CAD build for the part. Positions are in the model's coordinates, mm. Face numbers are marked on the shaded views. A direction names the side the tool comes from. Round coordinates to 2 decimals unless told otherwise and drop trailing zeros. Loops run counter-clockwise (first coordinate to the right, second up) from the corner with the lowest first, then second, coordinate; pieces in that order, holes last. Notation, with made-up numbers: (-34, 5.25) - (19, 5.25) arc R22 ccw to (19, 40.25) - close; hole circle Ø4 at (-0.5, -26). An arc over 180 degrees is marked (long way). One line per question, with ' | ' between items.
```python
from build123d import *

# Parameters (mm, degrees)
BASPROSKE_W              = 6
BASPROSKE_H              = 11.25
TOOTHCUT_DEPTH           = 18.003676073
TEETHCUTS_COUNT          = 16
TEETHCUTS_ANGLE          = 337.5
BORSKE_R                 = 0.4
BORE_DEPTH               = 50.0000508
TAGLIO_ESTRUSIONE1_DEPTH = 10


with BuildPart() as part:
    # BasProSke → Base-Revolve (revolve)
    with BuildSketch(Plane(origin=(0, 0, 0), x_dir=(1, 0, 0), z_dir=(0, 1, 0)), mode=Mode.PRIVATE) as base_revolve_sk:
        with Locations((3, 5.625)):
            Rectangle(BASPROSKE_W, BASPROSKE_H)
    revolve(base_revolve_sk.sketch.rotate(Axis((-10, 0, 0), (1, 0, 0)), 180), axis=Axis((-10, 0, 0), (1, 0, 0)))

    # TooCutSke → ToothCut (cut, through all)
    with BuildSketch(Plane(origin=(0, 0, 0), x_dir=(0, 0, -1), z_dir=(1, 0, 0))):
        with BuildLine():
            ThreePointArc((0.651061533, 8.411340626), (0, 8.4365), (-0.651061533, 8.411340626))
            ThreePointArc((-0.651061533, 8.411340626), (-1.029874156, 9.883978829), (-1.930926138, 11.108832945))
            ThreePointArc((-1.930926138, 11.108832945), (0, 11.2754), (1.930926138, 11.108832945))
            ThreePointArc((1.930926138, 11.108832945), (1.029874156, 9.883978829), (0.651061533, 8.411340626))
        make_face()
    toothcut = extrude(amount=TOOTHCUT_DEPTH, mode=Mode.SUBTRACT)

    # TeethCuts: ToothCut ×16 about axis
    teethcuts_axis = Axis((-10, 0, 0), (1, 0, 0))
    for i in range(1, TEETHCUTS_COUNT):
        add(toothcut.rotate(teethcuts_axis, i * TEETHCUTS_ANGLE / (TEETHCUTS_COUNT - 1)), mode=Mode.SUBTRACT)

    # BorSke → Bore (cut, symmetric)
    with BuildSketch(Plane(origin=(0, 0, 0), x_dir=(0, 0, -1), z_dir=(1, 0, 0))):
        with Locations(Location((0, 0, 0), (0, 0, 180))):
            Circle(BORSKE_R)
    extrude(amount=BORE_DEPTH, both=True, mode=Mode.SUBTRACT)

    # Schizzo1 → Taglio-Estrusione1 (cut)
    # profile 1 of 3: a face of its own
    with BuildSketch(Plane(origin=(6, 0, 0), x_dir=(0, 0, -1), z_dir=(1, 0, 0))):
        with BuildLine():
            ThreePointArc((1.5, 4.769696007), (0.758788496, 4.942088629), (0, 5))
            ThreePointArc((0, 5), (-0.758788496, 4.942088629), (-1.5, 4.769696007))
            ThreePointArc((-1.5, 4.769696007), (-2.958039892, -4.031128874), (5, 0))
            ThreePointArc((5, 0), (4.031128874, 2.958039892), (1.5, 4.769696007))
        make_face()
        with BuildLine():
            ThreePointArc((0.4, 0), (-0.282842712, -0.282842712), (0, 0.4))
            ThreePointArc((0, 0.4), (0.282842712, 0.282842712), (0.4, 0))
        make_face(mode=Mode.SUBTRACT)
    # profile 2 of 3: a face of its own
    with BuildSketch(Plane(origin=(6, 0, 0), x_dir=(0, 0, -1), z_dir=(1, 0, 0))):
        with BuildLine():
            ThreePointArc((-1.5, 4.769696007), (-0.758788496, 4.942088629), (0, 5))
            Line((0, 5), (0, 6.169696007))
            Line((0, 6.169696007), (-1.5, 6.169696007))
            Line((-1.5, 6.169696007), (-1.5, 4.769696007))
        make_face()
    # profile 3 of 3: a face of its own
    with BuildSketch(Plane(origin=(6, 0, 0), x_dir=(0, 0, -1), z_dir=(1, 0, 0))):
        with BuildLine():
            Line((0, 6.169696007), (0, 5))
            ThreePointArc((0, 5), (0.758788496, 4.942088629), (1.5, 4.769696007))
            Line((1.5, 4.769696007), (1.5, 6.169696007))
            Line((1.5, 6.169696007), (0, 6.169696007))
        make_face()
    extrude(amount=-TAGLIO_ESTRUSIONE1_DEPTH, mode=Mode.SUBTRACT)


solid = part.part
```
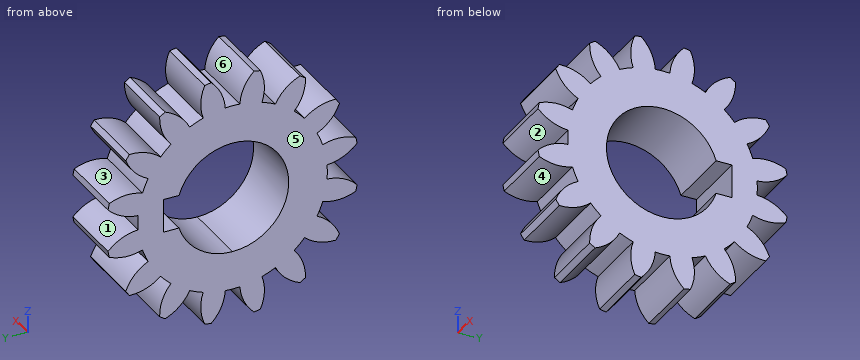
(1) Cut at C-C, the plane z = -7.25. Write the cut outline in (x, y).
Results found:
outline: (0, -6.06) - (6, -6.06) - (6, 6.06) - (0, 6.06) - close
(2) Drop flat-ended pins along their axis: P1, Ø0.7, axis at x = 4.5, y = 5, coming from the -Z side; P2, Ø3, axis at y = 6.5, z = -3.5, coming from the -X side; P3, Ø0.7, axis at x = 3, y = 5, coming from the +Z side; P4, Ø0.9, axis at x = 2, z = -0.5, coming from the -Y side. Give the stop position or say it passes through.
Results found:
P1: stops at z = -9.2 | P2: stops at x = 0 | P3: stops at z = 9.2 | P4: stops at y = -9.7
(3) Cut at A-A, the plane z = 0. Write the cut outline in (x, y), then the cut area to 3 significant figures.
Results found:
outline: (0, -8.44) - (6, -8.44) - (6, -5) - (0, -5) - close; (0, 6.17) - (6, 6.17) - (6, 8.44) - (0, 8.44) - close | area: 34.2 mm²
(4) Cut at B-B, the plane y = -3.5. Write the cut outline in (x, z), then the cut area to 3 significant figures.
Results found:
outline: (0, -7.68) - (6, -7.68) - (6, -3.57) - (0, -3.57) - close; (0, 3.57) - (6, 3.57) - (6, 7.68) - (0, 7.68) - close | area: 49.3 mm²
(5) Tool access for the marked faces 1, 2 and 3: list every direction of +Z, -Z, +X, -X, +Y, -Y with a clear straight run to the whole face (end or side of a thin tool).
Results found:
face 1: +X, -X, +Y | face 2: +X, -X, -Y | face 3: +X, -X
(6) Probe L1, parallel to Y at x = 5.2, z = 9; L2, parallel to Z at x = 3.3, y = 1.75; L3, parallel to Z at x = 4.4, y = 5.75. List the from-to ranges inside material, lowest first.
Results found:
L1: y = -6.49 to -5.06, -2.82 to -0.73, 0.73 to 2.82, 5.06 to 6.49 | L2: z = -10.93 to -4.68, 4.68 to 10.93 | L3: z = -9.41 to -6.74, -6.17 to -1.5, 1.5 to 6.17, 6.74 to 9.41
(7) Two-plate mould, pull along Z, no slides. Class the marked faces 4, 5 and 6: released by +Z, released by -Z, zero draft, split by the parting line, or undercut.
Results found:
face 4: undercut | face 5: zero draft | face 6: released by +Z
